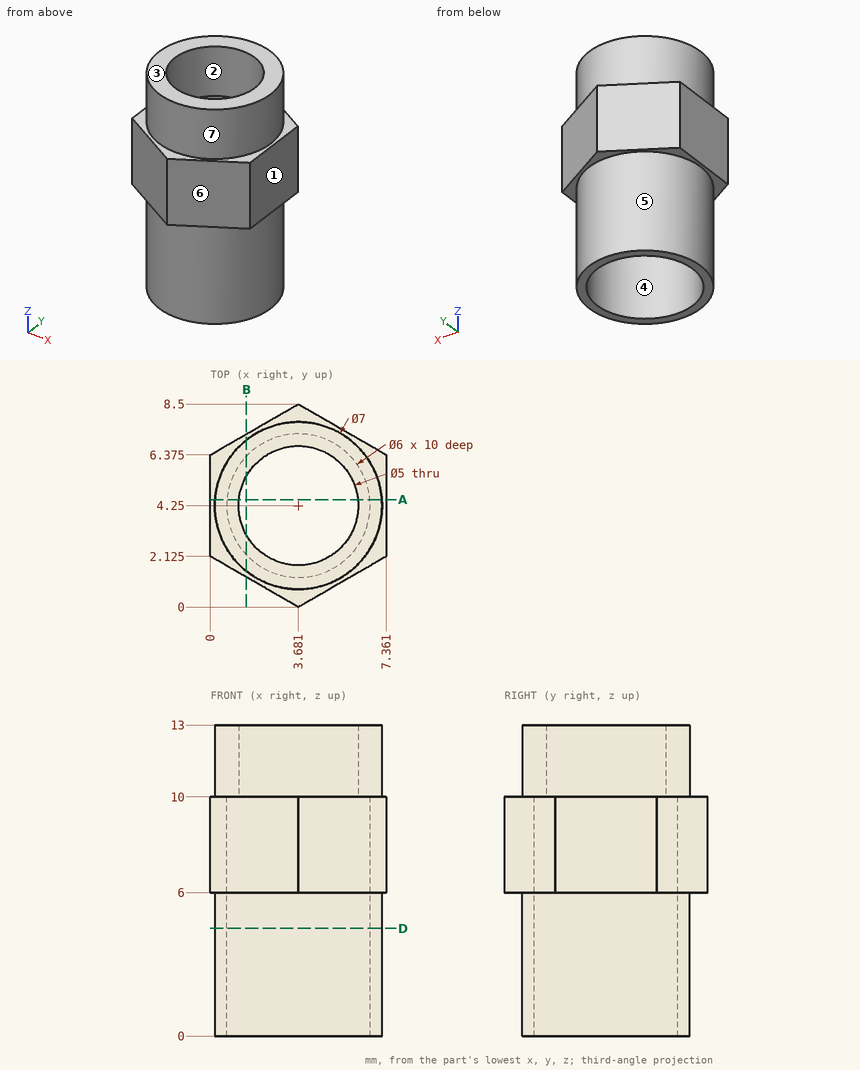
Job drawing, mm, ordinate dimensions from the low corner. One solid piece. A direction names the side the tool comes from. Coordinates: 2 decimals unless noted, no trailing zeros. Order: outer loops, then holes, each group sorted by start corner. A loop starts at its lowest first (then second) coordinate and runs counter-clockwise, first axis right, second up. Notation, with made-up numbers: (30.25, 77) -> (38.25, 77) arc R30 cw to (38.25, 103) -> close; hole circle Ø6 at (14, 55). An arc over 180 degrees is marked (long way). Answer in a Markdown table with one row per item. Add a question column.
Q1. Mould opens along X. For the marked faces 1, 2, 3 and 4 say: +X half, -X half, draft (parallel to the pull), parting line (faces both ways), or undercut.
Q2. Band-saw the part on B-B, the plane x = 1.5. List the corners of the cut face in (y, z).
Q3. Band-saw the part on D-D, the plane z = 4.5. List the corners of the cut face in (x, y), then the cut area to 3 significant figures.
Q4. Wall check: line 1 along X through (y, z) = (4.25, 7.5); line 2 along Z through (x, y) = (6.25, 6.75); line 3 along Z through (x, y) = (2.75, 7). Give the ranges that are in metal, low to high. Write a range as [from, to].
Q5. Which spindle directions (+Z, -Z, +X, -X, +Y, -Y) get a long thin tool onto all of the face, cutting with end or side? Do the marked faces 5, 6 and 7. Say none if no direction does.
Q6. Band-saw the part on A-A, the plane y = 4.5. List the corners of the cut face in (x, z).
Q7. Drop flat-ended pins along their axis: pin 1 (5 mm diameter, centred on y = 4.5, z = 2, fed in from +X); pin 2 (1.5 mm diameter, centred on x = 6.5, z = 1.5, fed in from -Y); pin 3 (1 mm diameter, centred on x = 4.5, z = 3, fed in from -Y) (1 decimal). Give the stop position or say it passes through.
Answers follow:
| question | item | result |
|---|---|---|
| 1 | face 1 | +X half |
| 1 | face 2 | undercut |
| 1 | face 3 | draft |
| 1 | face 4 | undercut |
| 2 | outline | (1.26, 6) -> (1.51, 6) -> (1.51, 0) -> (2.19, 0) -> (2.19, 10) -> (3.03, 10) -> (3.03, 13) -> (1.51, 13) -> (1.51, 10) -> (1.26, 10) -> close; (5.47, 10) -> (6.31, 10) -> (6.31, 0) -> (6.99, 0) -> (6.99, 6) -> (7.24, 6) -> (7.24, 10) -> (6.99, 10) -> (6.99, 13) -> (5.47, 13) -> close |
| 3 | outline | circle Ø7 at (3.68, 4.25); hole circle Ø6 at (3.68, 4.25) |
| 3 | area | 10.2 mm^2 |
| 4 | line 1 | [0, 0.68], [6.68, 7.36] |
| 4 | line 2 | [6, 10] |
| 4 | line 3 | [10, 13] |
| 5 | face 5 | -Z |
| 5 | face 6 | +Z, -Z, +X, -Y |
| 5 | face 7 | +Z |
| 6 | outline | (0, 6) -> (0.19, 6) -> (0.19, 0) -> (0.69, 0) -> (0.69, 10) -> (1.19, 10) -> (1.19, 13) -> (0.19, 13) -> (0.19, 10) -> (0, 10) -> close; (6.17, 10) -> (6.67, 10) -> (6.67, 0) -> (7.17, 0) -> (7.17, 6) -> (7.36, 6) -> (7.36, 10) -> (7.17, 10) -> (7.17, 13) -> (6.17, 13) -> close |
| 7 | pin 1 | x = 7.18 |
| 7 | pin 2 | y = 1.43 |
| 7 | pin 3 | y = 0.8 |
